```python
from build123d import *

# Parameters (mm, degrees)
SKETCH_2_W          = 49.3
SKETCH_2_H          = 38
SKETCH_2_R          = 1.75
SKETCH_2_W_2        = 13
SKETCH_2_H_2        = 10
EXTRUDE_1_DEPTH     = 30
FILLET_2_R          = 10
SKETCH_5_R          = 1.5
SKETCH_5_W          = 13
SKETCH_5_H          = 11.272014512
CUT_EXTRUDE_2_DEPTH = 20


with BuildPart() as part:
    # Эскиз2 → Бобышка-Вытянуть1 (new body)
    # profile 1 of 3: a face of its own
    with BuildSketch(Plane.XY):
        Rectangle(SKETCH_2_W, SKETCH_2_H)
        with Locations((-19.9, 1)):
            Circle(SKETCH_2_R, mode=Mode.SUBTRACT)
        with Locations((19.9, 1)):
            Circle(SKETCH_2_R, mode=Mode.SUBTRACT)
    # profile 2 of 3: a face of its own
    with BuildSketch(Plane.XY):
        with Locations((-31.15, -14)):
            Rectangle(SKETCH_2_W_2, SKETCH_2_H_2)
    # profile 3 of 3: a face of its own
    with BuildSketch(Plane.XY):
        with Locations((31.15, -14)):
            Rectangle(SKETCH_2_W_2, SKETCH_2_H_2)
    extrude(amount=EXTRUDE_1_DEPTH)

    # Скругление2
    fillet_2_edges = [part.edges().sort_by_distance(p)[0] for p in [
        (-24.65, 19, 15),
        (24.65, 19, 15),
    ]]
    fillet(fillet_2_edges, radius=FILLET_2_R)

    # Эскиз5 → Вырез-Вытянуть2 (cut)
    with BuildSketch(Plane(origin=(0, -9, 0), x_dir=(1, 0, 0), z_dir=(0, 1, 0))):
        with Locations(Location((-31.15, -4, 0), (0, 0, 180))):
            Circle(SKETCH_5_R)
        with Locations(Location((-31.15, -14.727985488, 0), (0, 0, 180))):
            Circle(SKETCH_5_R)
        with Locations(Location((31.15, -14.727985488, 0), (0, 0, 270))):
            Circle(SKETCH_5_R)
        with Locations(Location((31.15, -4, 0), (0, 0, 270))):
            Circle(SKETCH_5_R)
        with Locations((-31.15, -24.363992744)):
            Rectangle(SKETCH_5_W, SKETCH_5_H)
        with Locations((31.15, -24.363992744)):
            Rectangle(SKETCH_5_W, SKETCH_5_H)
    extrude(amount=-CUT_EXTRUDE_2_DEPTH, mode=Mode.SUBTRACT)


solid = part.part
```
Design review of the part built by this model. Coordinates are the model's own, in mm. A direction names the side the tool comes from. Coordinates: 2 decimals unless noted, no trailing zeros. Order: outer loops, then holes, each group sorted by start corner. A loop starts at its lowest first (then second) coordinate and runs counter-clockwise, first axis right, second up.
1) Mouldability with a two-part tool opening along Y and no side actions: class faces 1 (the cylindrical face through (18.15, 1.08, 14.79)), 2 (the cylindrical face through (-32.58, -13.93, 4.45)), 3 (the cylindrical face through (21.64, 16.15, 15.21)) as +Y half, -Y half, draft (parallel to the pull), parting line (faces both ways), or undercut.
2) Take a section at D-D, the plane x = -20.5. Give the boundary of the cut face in (y, z), and give its area (3 significant figures).
3) Take a section at B-B, the plane x = 31.15. Give the boundary of the cut face in (y, z).
4) Take a section at C-C, the plane z = 21. Give the boundary of the cut face in (x, y).
5) Take a section at A-A, the plane y = 1. Give the boundary of the cut face in (x, z), and give its area (3 significant figures).
6) Wall thickness on line 1 along Z through (x, y) = (-31.15, -15.5); line 2 along X through (y, z) = (8, 24); line 3 along Y through (x, z) = (-19, 14.25): over which ranges is each line inside the solid? List them lowest first.
7) Clearance check with flat-ended pins moving along their axes: pin 1 (4 mm diameter, centred on x = 32, z = 9, fed in from +Y); pin 2 (5 mm diameter, centred on x = 30.5, y = -13.5, fed in from +Z); pin 3 (2 mm diameter, centred on y = -1.5, z = 11, fed in from -X); pin 4 (2 mm diameter, centred on x = -19.9, y = 1, fed in from -Z). State where each tip first meets the part, or that it passes through.
8) For faces 4 (the flat face through (31, -9, 9)), 5 (the flat face through (31, -14, 18.728)), 6 (the flat face through (-31, -9, 9)), 7 (the flat face through (-31, -14, 18.728)), list the 3-axis set-ups (+Z, -Z, +X, -X, +Y, -Y) from which the entire face can be reached by the end or side of a thin tool; tool diameter is ignored.
Returned:
1. face 1: undercut
1. face 2: draft
1. face 3: +Y half
2. outline: (-19, 0) - (-0.64, 0) - (-0.64, 30) - (-19, 30) - close; (2.64, 0) - (17.11, 0) - (17.11, 30) - (2.64, 30) - close
2. area: 985 mm2
3. outline: (-19, 0) - (-9, 0) - (-9, 2.5) - (-19, 2.5) - close; (-19, 5.5) - (-9, 5.5) - (-9, 13.23) - (-19, 13.23) - close; (-19, 16.23) - (-9, 16.23) - (-9, 18.73) - (-19, 18.73) - close
4. outline: (-24.65, -19) - (24.65, -19) - (24.65, 9) arc R10 ccw to (14.65, 19) - (-14.65, 19) arc R10 ccw to (-24.65, 9) - close; hole circle Ø3.5 at (-19.9, 1); hole circle Ø3.5 at (19.9, 1)
5. outline: (-24.65, 0) - (-21.65, 0) - (-21.65, 30) - (-24.65, 30) - close; (-18.15, 0) - (18.15, 0) - (18.15, 30) - (-18.15, 30) - close; (21.65, 0) - (24.65, 0) - (24.65, 30) - (21.65, 30) - close
5. area: 1,270 mm2
6. line 1: z = 0 to 2.5, 5.5 to 13.23, 16.23 to 18.73
6. line 2: x = -24.65 to 24.65
6. line 3: y = -19 to -0.5, 2.5 to 18
7. pin 1: stops at y = -9
7. pin 2: stops at z = 18.73
7. pin 3: stops at x = -24.65
7. pin 4: passes through
8. face 4: +Z, -Z, +X, +Y
8. face 5: +Z, +X, +Y, -Y
8. face 6: +Z, -Z, -X, +Y
8. face 7: +Z, -X, +Y, -Y
